```python
from build123d import *

# Parameters (mm, degrees)
SKETCH1_W           = 82.5
SKETCH1_H           = 46.5
SKETCH1_R           = 2.05
BOSS_EXTRUDE1_DEPTH = 4.5
SKETCH2_R           = 1.25
CUT_EXTRUDE1_DEPTH  = 5.5
SKETCH3_W           = 4.5
SKETCH3_H           = 4.5
CUT_EXTRUDE2_DEPTH  = 5.5


with BuildPart() as part:
    # Sketch1 → Boss-Extrude1 (new body)
    with BuildSketch(Plane(origin=(0, 0, 0), x_dir=(1, 0, 0), z_dir=(0, 1, 0))):
        Rectangle(SKETCH1_W, SKETCH1_H)
        with Locations((20.92918, 0)):
            Circle(SKETCH1_R, mode=Mode.SUBTRACT)
        with Locations((-10.07082, 0)):
            Circle(SKETCH1_R, mode=Mode.SUBTRACT)
    extrude(amount=BOSS_EXTRUDE1_DEPTH)

    # Sketch2 → Cut-Extrude1 (cut, through all)
    with BuildSketch(Plane(origin=(0, 4.5, 0), x_dir=(1, 0, 0), z_dir=(0, 1, 0))):
        with Locations((-31.25, -13.25)):
            Circle(SKETCH2_R)
        with Locations((-31.25, 13.25)):
            Circle(SKETCH2_R)
    extrude(amount=-CUT_EXTRUDE1_DEPTH, mode=Mode.SUBTRACT)

    # Sketch3 → Cut-Extrude2 (cut, through all)
    with BuildSketch(Plane(origin=(0, 0, 0), x_dir=(-1, 0, 0), z_dir=(0, -1, 0))):
        with Locations((34.5, 21)):
            Rectangle(SKETCH3_W, SKETCH3_H)
        with Locations((39, 4.5)):
            Rectangle(SKETCH3_W, SKETCH3_H)
        with Locations((39, -16.5)):
            Rectangle(SKETCH3_W, SKETCH3_H)
        with Locations((22.5, -21)):
            Rectangle(SKETCH3_W, SKETCH3_H)
        with Locations((1.5, -21)):
            Rectangle(SKETCH3_W, SKETCH3_H)
        with Locations((13.5, 21)):
            Rectangle(SKETCH3_W, SKETCH3_H)
    extrude(amount=-CUT_EXTRUDE2_DEPTH, mode=Mode.SUBTRACT)


solid = part.part
```
Design review of the part built by this model. Coordinates are the model's own, in mm. A direction names the side the tool comes from. Coordinates: 2 decimals unless noted, no trailing zeros. Order: outer loops, then holes, each group sorted by start corner. A loop starts at its lowest first (then second) coordinate and runs counter-clockwise, first axis right, second up. Notation, with made-up numbers: (3, 75) -> (53, 75) arc R15 ccw to (53, 82) -> close; hole circle Ø1 at (-20.75, 75.5). An arc over 180 degrees is marked (long way). One line per item, written item: value. Start each with the question number.
Q1. Take a section at B-B, the plane z = -13.25. State the section outline as (x, y) points, then the cut area to 3 significant figures.
Q2. Take a section at C-C, the plane z = 0. State the section outline as (x, y) points.
Q3. Insertion check: pin 1 Ø5.5 at (x, z) = (-10.07, 0) entering from -Y; pin 2 Ø2 at (y, z) = (2, 17) entering from -X; pin 3 Ø1.3 at (x, y) = (-21.5, 1.5) entering from +Z; pin 4 Ø2 at (x, y) = (-14, 1.5) entering from -Z. Each pin has a flat end and moves straight along its axis. Give the tip position at first contact, or say it passes through.
Q4. Tool access review of faces 1 (the flat face through (-22, 2, 18.75)), 2 (the flat face through (-1, 0, 0)), 3 (the flat face through (-39, 2, -2.25)), 4 (the flat face through (-11.25, 2, -21)): name each direction out of +Z, -Z, +X, -X, +Y, -Y from which nothing blocks a thin tool from reaching the whole face with its end or side.
Q5. Take a section at D-D, the plane y = 3.4. Give the number of separate pieces and of enclosed holes in the cut face, then the cut area to 3 significant figures.
Q6. Take a section at A-A, the plane x = -31.25. State the section outline as (y, z) points, then the cut area to 3 significant figures.
Q7. Mouldability with a two-part tool opening along X and no side actions: class faces 5 (the flat face through (-36.75, 2, 17)), 6 (the flat face through (-39, 2, -6.75)), 7 (the flat face through (-3.75, 2, 21)) as pulls with the +X half, pulls with the -X half, needs draft (parallel to the pull), parting line crosses it, or undercut.
Q8. For probe 1 along X at (y, z) = (1.1, 0); probe 2 along Z at (x, y) = (-31.25, 1.3); probe 3 along X at (y, z) = (1.5, -13.25), list the stretches that pass through material, from the lowest coordinate up.
Values follow:
1. outline: (-41.25, 0) -> (-32.5, 0) -> (-32.5, 4.5) -> (-41.25, 4.5) -> close; (-30, 0) -> (41.25, 0) -> (41.25, 4.5) -> (-30, 4.5) -> close
1. area: 360 mm2
2. outline: (-41.25, 0) -> (-12.12, 0) -> (-12.12, 4.5) -> (-41.25, 4.5) -> close; (-8.02, 0) -> (18.88, 0) -> (18.88, 4.5) -> (-8.02, 4.5) -> close; (22.98, 0) -> (41.25, 0) -> (41.25, 4.5) -> (22.98, 4.5) -> close
3. pin 1: stops at y = 0
3. pin 2: stops at x = -36.75
3. pin 3: stops at z = 18.75
3. pin 4: stops at z = -18.75
4. face 1: +Z, +Y, -Y
4. face 2: +Z, -Z, +X, -X, -Y
4. face 3: -X, +Y, -Y
4. face 4: -Z, +Y, -Y
5. separate pieces: 1
5. enclosed holes: 4
5. area: 3,680 mm2
6. outline: (0, -23.25) -> (4.5, -23.25) -> (4.5, -14.5) -> (0, -14.5) -> close; (0, -12) -> (4.5, -12) -> (4.5, 12) -> (0, 12) -> close; (0, 14.5) -> (4.5, 14.5) -> (4.5, 23.25) -> (0, 23.25) -> close
6. area: 187 mm2
7. face 5: pulls with the -X half
7. face 6: needs draft
7. face 7: undercut
8. probe 1: x = -41.25 to -12.12, -8.02 to 18.88, 22.98 to 41.25
8. probe 2: z = -23.25 to -14.5, -12 to 12, 14.5 to 23.25
8. probe 3: x = -41.25 to -32.5, -30 to 41.25
